```python
from build123d import *

# Parameters (mm, degrees)
F1_DEPTH = 25
F2_R     = 5


with BuildPart() as f1:
    # F0 (on Top) → F1 (new body)
    with BuildSketch(Plane.XY):
        with BuildLine():
            Line((73.27253, 59.831257), (-89.452814, 59.831257))
            ThreePointArc((-89.452814, 59.831257), (-96.523882, 56.902325), (-99.452814, 49.831257))
            Line((-99.452814, 49.831257), (-99.452814, -50.168743))
            ThreePointArc((-99.452814, -50.168743), (-96.523882, -57.239811), (-89.452814, -60.168743))
            Line((-89.452814, -60.168743), (72.86438, -60.168743))
            ThreePointArc((72.86438, -60.168743), (85.371822, -55.775277), (92.384161, -44.525133))
            ThreePointArc((92.384161, -44.525133), (45.345589, 0.480687), (92.488089, 45.377633))
            ThreePointArc((92.488089, 45.377633), (85.294852, 55.814491), (73.27253, 59.831257))
        make_face()
    extrude(amount=F1_DEPTH)

    # F2
    f2_edges = [f1.edges().sort_by_distance(p)[0] for p in [
        (-8.090142, 59.831257, 25),
        (-99.452814, -0.168743, 25),
        (-8.294217, -60.168743, 25),
        (45.345589, 0.480687, 25),
    ]]
    fillet(f2_edges, radius=F2_R)


solid = f1.part
```
Design review of the part built by this model. Coordinates are the model's own, in mm. Coordinates: 2 decimals unless noted, no trailing zeros. Loops run counter-clockwise (first coordinate to the right, second up) from the corner with the lowest first, then second, coordinate; pieces in that order, holes last. Notation, with made-up numbers: (70, -22) - (119, -22) arc R16 ccw to (119, 1) - close; hole circle Ø8 at (55.25, 3.25). An arc over 180 degrees is marked (long way). Use CSV: the item, a comma, the result in double quotes. Start each with the question number.
1) For pin 1 Ø1 at (x, y) = (64.5, 35.5) entering from +Z, flat-tipped, find the tip position at first contact; note if it passes through.
2) Consider section A-A on z = 18. Write out the cut boundary in (x, y).
3) Wall thickness on L1, parallel to X at y = 54, z = 3; L2, parallel to Y at x = -77, z = 22.5; L3, parallel to Y at x = -77.5, z = 23: over which ranges is each line inside the solid? List them lowest first. Write a range as from..to.
Geometry says:
1,pin 1,"through"
2,outline,"(-99.45, -50.17) arc R10 ccw to (-89.45, -60.17) - (72.86, -60.17) arc R20 ccw to (92.38, -44.53) arc R45 cw (long way) to (92.49, 45.38) arc R20 ccw to (73.27, 59.83) - (-89.45, 59.83) arc R10 ccw to (-99.45, 49.83) - close"
3,L1,"-98.54..87.39"
3,L2,"-59.5..59.16"
3,L3,"-59.17..58.83"
